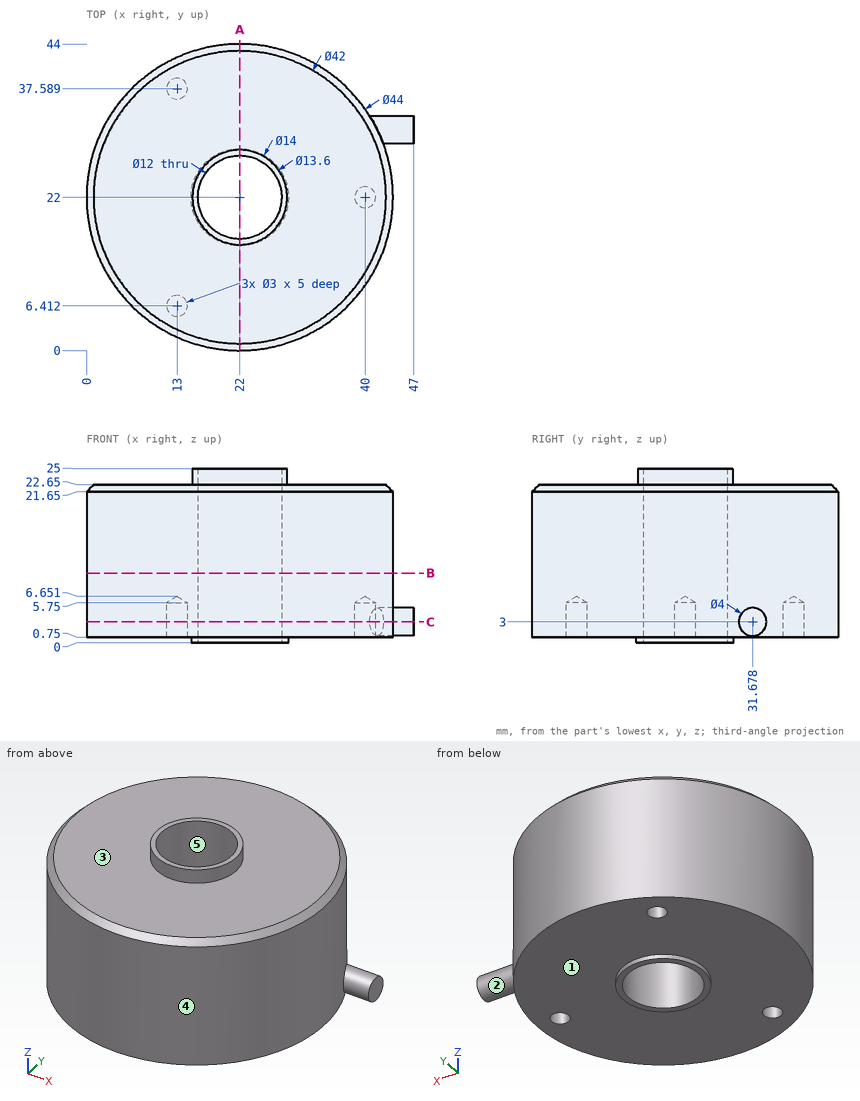
Input: dimensioned drawing with shaded views. Units: mm. Origin: part minimum x, y, z. A direction names the side the tool comes from. Round coordinates to 2 decimals unless told otherwise and drop trailing zeros. Loops run counter-clockwise (first coordinate to the right, second up) from the corner with the lowest first, then second, coordinate; pieces in that order, holes last. Notation, with made-up numbers: M 70,44 L 76,44 A23 cw 76,64 Z; hole C 45,13 d7. An arc over 180 degrees is marked long. Return JSON: item names as keys, results as strings. Group by question number.
1. Section query A-A on x = 22. Output: boundary loops of the cut face in (y, z).
2. Pin query (flat end, axial travel): pin 1 (3 mm diameter, centred on y = 38, z = 6, fed in from +X) (1 decimal); pin 2 (2.5 mm diameter, centred on x = 40, y = 22, fed in from -Z); pin 3 (8 mm diameter, centred on x = 14.5, y = 5.5, fed in from -Z); pin 4 (9.5 mm diameter, centred on x = 22, y = 22, fed in from -Z). Return the tip coordinate at first contact, or that it passes through.
3. Mould query, pull axis X, two halves, no side actions, for the marked faces 3, 4 and 5. Classes: released by +X, released by -X, zero draft, split by the parting line, or undercut.
4. Section query C-C on z = 3. Output: boundary loops of the cut face in (x, y) (1 decimal), and give its area (3 significant figures).
5. Material intervals for line 1 along Z through (x, y) = (28.5, 27.5); line 2 along X through (y, z) = (18.5, 17) (1 decimal); line 3 along X through (y, z) = (20.5, 21.25), sorted ascending. Write a range as from..to.
6. Section query B-B on z = 10. Output: boundary loops of the cut face in (x, y).
7. Reachability of the marked faces 1 and 2 from +Z, -Z, +X, -X, +Y, -Y: full face, straight path, thin tool, end or side. Return the list, or none.
Checks:
{
 "1": {"outline": "M 0,0.75 L 15,0.75 L 15,0 L 16,0 L 16,25 L 15.2,25 L 15.2,22.65 L 1,22.65 L 0,21.65 Z; M 28,0 L 29,0 L 29,0.75 L 44,0.75 L 44,21.65 L 43,22.65 L 28.8,22.65 L 28.8,25 L 28,25 Z"},
 "2": {"pin 1": "stops at x = 38.5", "pin 2": "stops at z = 5.9", "pin 3": "stops at z = 0.75", "pin 4": "passes through"},
 "3": {"face 3": "zero draft", "face 4": "split by the parting line", "face 5": "undercut"},
 "4": {"outline": "M 40.6,33.7 A22 ccw long 42.6,29.7 L 47,29.7 L 47,33.7 Z; hole C 13,6.4 d3; hole C 13,37.6 d3; hole C 22,22 d12; hole C 40,22 d3", "area": "1,410 mm²"},
 "5": {"line 1": "z = 0.75..22.65", "line 2": "x = 0.3..17.1, 26.9..43.7", "line 3": "x = 0.05..16.19, 27.81..43.95"},
 "6": {"outline": "C 22,22 d44; hole C 22,22 d12"},
 "7": {"face 1": "-Z", "face 2": "+X"}
}
